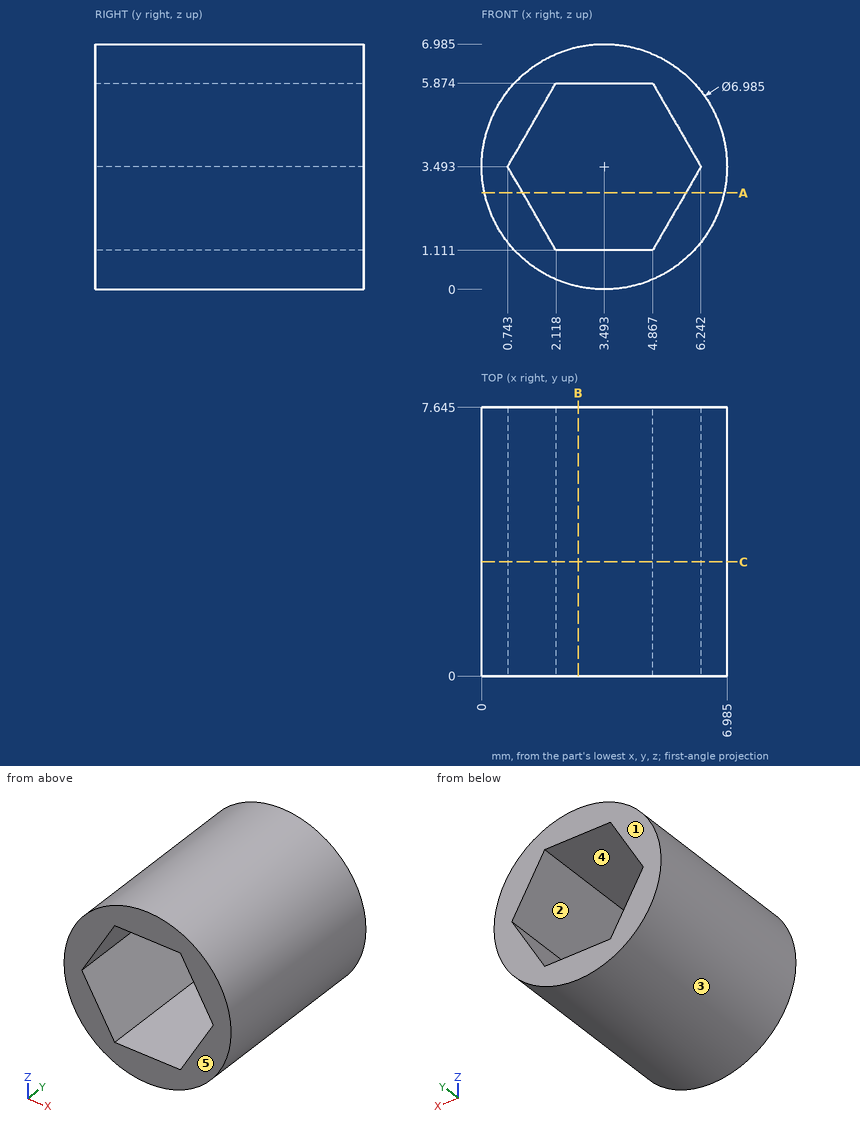
Study the drawing (mm; zero at the part's minimum x, y, z) and answer. A direction names the side the tool comes from. Give positions to 0.01 mm unless a question says otherwise; leave off trailing zeros. Loops run counter-clockwise (first coordinate to the right, second up) from the corner with the lowest first, then second, coordinate; pieces in that order, holes last. Notation, with made-up numbers: (47.5, 87.5) - (75.5, 87.5) arc R16 ccw to (75.5, 93.5) - close; hole circle Ø3 at (82, 43). An arc over 180 degrees is marked (long way). One line per question, with ' | ' between items.
(1) Straight lines are drawn through the part: probe 1 along Z at (x, y) = (5.75, 6.75) (1 decimal); probe 2 along Z at (x, y) = (3.75, 3.5) (1 decimal); probe 3 along X at (y, z) = (6.5, 1.5) (1 decimal). For each, find the intervals that lie inside material, in ascending order.
Recorded:
probe 1: z = 0.8 to 2.6, 4.3 to 6.2 | probe 2: z = 0 to 1.1, 5.9 to 7 | probe 3: x = 0.6 to 1.9, 5.1 to 6.4
(2) The mould has two halves that part along Z. Classify the marked faces 1, 2 and 3: +Z half, -Z half, draft (parallel to the pull), parting line (faces both ways), or undercut.
Recorded:
face 1: draft | face 2: undercut | face 3: parting line
(3) The part is cut by section A-A (z = 2.75). Write down the section's boundary in (x, y) (1 decimal), then the cut area to 3 significant figures.
Recorded:
outline: (0.1, 0) - (1.2, 0) - (1.2, 7.6) - (0.1, 7.6) - close; (5.8, 0) - (6.9, 0) - (6.9, 7.6) - (5.8, 7.6) - close | area: 16.7 mm²
(4) A tool of negligible diameter and unlimited length cuts with its end or side. For the marked faces 4 and 5, from which of +Z, -Z, +X, -X, +Y, -Y can it reach the whole face along a straight path? Write none if from no direction.
Recorded:
face 4: +Y, -Y | face 5: +Z, -Z, +X, -X, -Y
(5) Each of these flat-tipped pins is pushed along its axis until it touches: pin 1 Ø4 at (y, z) = (2.5, 1.5) entering from +X (1 decimal); pin 2 Ø1 at (y, z) = (5.5, 2) entering from +X. Where does it stop, or does it pass through?
Recorded:
pin 1: stops at x = 7 | pin 2: stops at x = 6.84
(6) The part is cut by section B-B (x = 2.75). Write down the section's boundary in (y, z) (1 decimal).
Recorded:
outline: (0, 0.1) - (7.6, 0.1) - (7.6, 1.1) - (0, 1.1) - close; (0, 5.9) - (7.6, 5.9) - (7.6, 6.9) - (0, 6.9) - close
(7) The part is cut by section C-C (y = 3.25). Write down the section's boundary in (x, z) (1 decimal).
Recorded:
outline: circle Ø7 at (3.5, 3.5); hole (0.7, 3.5) - (2.1, 1.1) - (4.9, 1.1) - (6.2, 3.5) - (4.9, 5.9) - (2.1, 5.9) - close
